Input: part model. Units: mm. Frame: model coordinates. A direction names the side the tool comes from. Give positions to 0.01 mm unless a question says otherwise; leave off trailing zeros. Write each loop counter-clockwise with the first axis right and the second up, starting at its lowest first coordinate (ties: lowest second). Pieces come first, ordered by that corner, then holes. Notation, with made-up numbers: (57.5, 43.5) - (91.5, 43.5) arc R28 cw to (91.5, 67.5) - close; hole circle Ø10 at (56.25, 52.25). An arc over 180 degrees is marked (long way). Answer as CSV lines item,"result". Start each with the question number.
from build123d import *

# Parameters (mm, degrees)
SKETCH2_W           = 40
SKETCH2_H           = 10
BOSS_EXTRUDE1_DEPTH = 4
SKETCH3_R           = 1
CUT_EXTRUDE1_DEPTH  = 22
SKETCH4_R           = 2
CUT_EXTRUDE2_DEPTH  = 2


with BuildPart() as part:
    # Sketch2 → Boss-Extrude1 (new body)
    with BuildSketch(Plane.XY):
        Rectangle(SKETCH2_W, SKETCH2_H)
    extrude(amount=BOSS_EXTRUDE1_DEPTH)

    # Sketch3 → Cut-Extrude1 (cut, through all)
    with BuildSketch(Plane.XY.offset(4)):
        with Locations((-17, 3.2)):
            Circle(SKETCH3_R)
        with Locations((0, 3.2)):
            Circle(SKETCH3_R)
        with Locations((17, 3.2)):
            Circle(SKETCH3_R)
        with Locations((-7.5, -2)):
            Circle(SKETCH3_R)
        with Locations((7.5, -2)):
            Circle(SKETCH3_R)
    extrude(amount=-CUT_EXTRUDE1_DEPTH, mode=Mode.SUBTRACT)

    # Sketch4 → Cut-Extrude2 (cut)
    with BuildSketch(Plane.XY.offset(4)):
        with Locations((-7.5, -2)):
            Circle(SKETCH4_R)
        with Locations((7.5, -2)):
            Circle(SKETCH4_R)
    extrude(amount=-CUT_EXTRUDE2_DEPTH, mode=Mode.SUBTRACT)


solid = part.part
1) Cut plane C-C on x = -17. Output: boundary loops of the cut face in (y, z), and give its area (3 significant figures).
2) Contact query for flat-ended pins moving along their axis: P1, Ø1.8, axis at x = -17, y = 3.2, coming from the -Z side; P2, Ø2.5, axis at x = -7.5, y = -2, coming from the +Z side. Output: stop coordinate, or through.
3) Pull-direction query (Y, two-part tool) for faces 3 (the cylindrical face through (-9.498, -1.912, 3.014)), 4 (the flat face through (0, -5, 2)), 5 (the flat face through (20, 0, 2)); classes: +Y half, -Y half, draft (parallel to the pull), parting line (faces both ways), or undercut.
4) Reachability of faces 1 (the flat face through (0, 5, 2)), 2 (the flat face through (8.4, -2.9, 2)) from +Z, -Z, +X, -X, +Y, -Y: full face, straight path, thin tool, end or side. Return the list, or none.
5) Material intervals for line 1 (X direction, y = -3, z = 2.75); line 2 (X direction, y = -3.75, z = 3.1); line 3 (X direction, y = 3.5, z = 2.8), sorted ascending. Write a range as from..to.
6) Cut plane D-D on x = -7.5. Output: boundary loops of the cut face in (y, z).
7) Cut plane B-B on z = 1.4. Output: boundary loops of the cut face in (x, y), and give its area (3 significant figures).
8) Cut plane A-A on y = 3.2. Output: boundary loops of the cut face in (x, z).
Numbers:
1,outline,"(-5, 0) - (2.2, 0) - (2.2, 4) - (-5, 4) - close; (4.2, 0) - (5, 0) - (5, 4) - (4.2, 4) - close"
1,area,"32.0 mm²"
2,P1,"passes through"
2,P2,"stops at z = 2"
3,face 3,"undercut"
3,face 4,"-Y half"
3,face 5,"draft"
4,face 1,"+Z, -Z, +X, -X, +Y"
4,face 2,"+Z"
5,line 1,"x = -20..-9.23, -5.77..5.77, 9.23..20"
5,line 2,"x = -20..-8.47, -6.53..6.53, 8.47..20"
5,line 3,"x = -20..-17.95, -16.05..-0.95, 0.95..16.05, 17.95..20"
6,outline,"(-5, 0) - (-3, 0) - (-3, 2) - (-4, 2) - (-4, 4) - (-5, 4) - close; (-1, 0) - (5, 0) - (5, 4) - (0, 4) - (0, 2) - (-1, 2) - close"
7,outline,"(-20, -5) - (20, -5) - (20, 5) - (-20, 5) - close; hole circle Ø2 at (-17, 3.2); hole circle Ø2 at (-7.5, -2); hole circle Ø2 at (0, 3.2); hole circle Ø2 at (7.5, -2); hole circle Ø2 at (17, 3.2)"
7,area,"384 mm²"
8,outline,"(-20, 0) - (-18, 0) - (-18, 4) - (-20, 4) - close; (-16, 0) - (-1, 0) - (-1, 4) - (-16, 4) - close; (1, 0) - (16, 0) - (16, 4) - (1, 4) - close; (18, 0) - (20, 0) - (20, 4) - (18, 4) - close"
